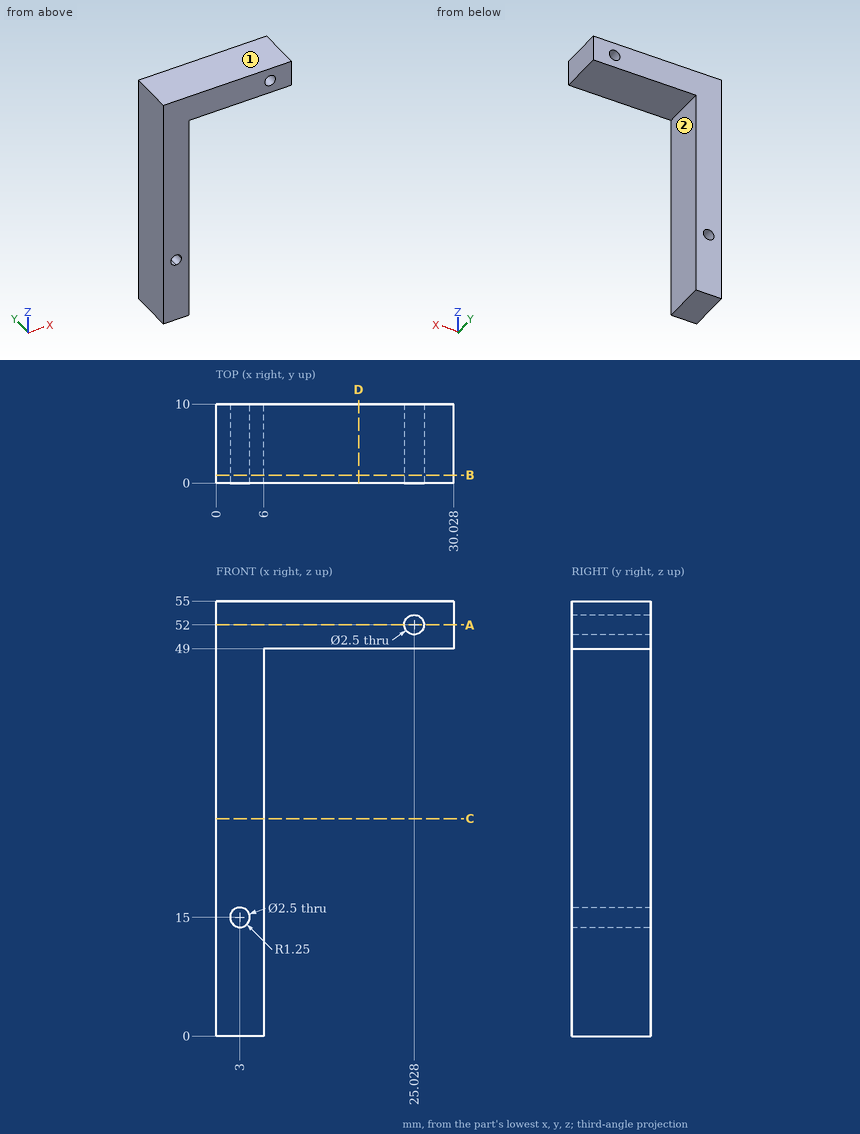
Geometry check sheet. Reference: drawing and pictorial views, mm from the part's lowest x, y, z. A direction names the side the tool comes from. Round coordinates to 2 decimals unless told otherwise and drop trailing zeros. Loops run counter-clockwise (first coordinate to the right, second up) from the corner with the lowest first, then second, coordinate; pieces in that order, holes last. Notation, with made-up numbers: (35.5, 55) - (45.5, 55) arc R17 ccw to (45.5, 84) - close; hole circle Ø7 at (53, 6). An arc over 180 degrees is marked (long way). Answer in a Markdown table with one row per item. Add a question column.
Q1. Gauge pin test, flat ends, axial feed: pin 1 (6 mm diameter, centred on y = 6.5, z = 8.5, fed in from +X); pin 2 (4 mm diameter, centred on y = 7.5, z = 39.5, fed in from -X); pin 3 (2 mm diameter, centred on x = 24, y = 3, fed in from -Z). Record the tip position at first contact, or that the pin passes through.
Q2. Tool access check on the marked faces 1 and 2. Record the directions out of +Z, -Z, +X, -X, +Y, -Y that give a thin tool (end or side, any length) a straight path to the whole face; none if there is none.
Q3. Material ranges on line 1 (Z direction, x = 3, y = 4.5); line 2 (X direction, y = 4, z = 15); line 3 (X direction, y = 9.25, z = 41), recorded low to high.
Q4. Section check B-B on y = 1. Enter the section's corners in (x, z), plus the area to 3 significant figures.
Q5. Section check D-D on x = 18. Enter the section's corners in (y, z).
Q6. Section check C-C on z = 27.5. Enter the section's corners in (x, y).
Q7. Section check A-A on z = 52. Enter the section's corners in (x, y).
Found:
| question | item | result |
|---|---|---|
| 1 | pin 1 | stops at x = 6 |
| 1 | pin 2 | stops at x = 0 |
| 1 | pin 3 | stops at z = 49 |
| 2 | face 1 | +Z, +X, -X, +Y, -Y |
| 2 | face 2 | -Z, +X, +Y, -Y |
| 3 | line 1 | z = 0 to 13.75, 16.25 to 55 |
| 3 | line 2 | x = 0 to 1.75, 4.25 to 6 |
| 3 | line 3 | x = 0 to 6 |
| 4 | outline | (0, 0) - (6, 0) - (6, 49) - (30.03, 49) - (30.03, 55) - (0, 55) - close; hole circle Ø2.5 at (3, 15); hole circle Ø2.5 at (25.03, 52) |
| 4 | area | 464 mm² |
| 5 | outline | (0, 49) - (10, 49) - (10, 55) - (0, 55) - close |
| 6 | outline | (0, 0) - (6, 0) - (6, 10) - (0, 10) - close |
| 7 | outline | (0, 0) - (23.78, 0) - (23.78, 10) - (0, 10) - close; (26.28, 0) - (30.03, 0) - (30.03, 10) - (26.28, 10) - close |
